Source: CAD feature listing. Evaluate the final solid. Frame: model axes, mm. A direction names the side the tool comes from. Give positions to 0.01 mm unless a question says otherwise; leave off trailing zeros. Loops run counter-clockwise (first coordinate to the right, second up) from the corner with the lowest first, then second, coordinate; pieces in that order, holes last. Notation, with made-up numbers: (-16.5, 25.25) -> (34.5, 25.25) arc R21 ccw to (34.5, 61.25) -> close; hole circle Ø9 at (-23.5, 60.25). An arc over 180 degrees is marked (long way). Put each result on its own line as item: value.
Autodesk Inventor part; units mm, degrees
ref_plane "YZ Plane" through (0, 0, 0) normal (1, 0, 0) x (0, 1, 0)
ref_plane "XZ Plane" through (0, 0, 0) normal (0, 1, 0) x (-1, 0, 0)
ref_plane "XY Plane" through (0, 0, 0) normal (0, 0, 1) x (1, 0, 0)
sketch "Sketch2" plane through (0, 0, 0) normal (0, 0, 1) x (1, 0, 0)
  circle A0 centre (0, 0) radius 14
  dimension "d1" = 28
extrude "Extrusion1" add sketch "Sketch2" along normal mid plane 30
sketch "Sketch3" plane through (0, 0, 15) normal (0, 0, 1) x (1, 0, 0)
  point P0 (0, 0)
hole "Hole1" at (0, 0, 15) direction (0, 0, -1) diameter 3.2 depth 5
sketch "Sketch4" plane through (0, 0, 10) normal (0, 0, 1) x (1, 0, 0)
  circle A0 centre (0, 0) radius 1.6
  line L0 (-1.5877, 2.75) -> (1.5877, 2.75)
  line L1 (1.5877, 2.75) -> (3.1754, 0)
  line L2 (3.1754, 0) -> (1.5877, -2.75)
  line L3 (1.5877, -2.75) -> (-1.5877, -2.75)
  line L4 (-1.5877, -2.75) -> (-3.1754, 0)
  line L5 (-3.1754, 0) -> (-1.5877, 2.75)
  dimension "d11" = 5.5
extrude "Extrusion2" cut sketch "Sketch4" against normal up to surface (10 mm away) contours A0 | L0 L1 L2 L3 L4 L5
sketch "Sketch5" plane through (0, 0, -15) normal (0, 0, -1) x (-1, 0, 0)
  circle A0 centre (0, 0) radius 2.5
  line L0 (-1.5, 2) -> (1.5, 2)
  dimension "d41" = 5
  dimension "d42" = 4.5
extrude "Extrusion3" cut sketch "Sketch5" against normal up to surface (15 mm away) contours A0 L0 picked at (0.1119, 0.5076)
sketch "Sketch8" plane through (0, 0, 0) normal (1, 0, 0) x (0, 1, 0)
  line L0 (2.85, 0) -> (-2.85, 0)
  line L1 (-2.85, 0) -> (-2.85, 2.6)
  line L2 (-2.85, 2.6) -> (2.85, 2.6)
  line L3 (2.85, 2.6) -> (2.85, 0)
  point P0 (0, 0)
  dimension "d48" = 2.6
  dimension "d49" = 5.7
extrude "Extrusion4" cut sketch "Sketch8" along normal through all both and the other way through all
equation "\"d30\" = 55deg"
equation "\"Sketch6_Pitch\" = 1.25"
properties part number "DestinationSpoolHolder"
(1) Line query: probe 1 along Z at (x, y) = (11, -2.75); probe 2 along X at (y, z) = (0, 13). Output: solid intervals per line, ascending. Write a range as from..to.
Calculated:
probe 1: z = -15..0, 2.6..15
probe 2: x = -14..-1.6, 1.6..14
(2) First-contact query: P1, Ø2, axis at y = 9, z = -4.5, coming from the +X side; P2, Ø12, axis at y = -7, z = 1.5, coming from the -X side; P3, Ø1, axis at x = 1.5, z = -2.5, coming from the +Y side; P4, Ø2.5, axis at x = 0, y = 0, coming from the +Z side. Flat tips, straight axial feed; report the tip coordinate or a pass-through.
Calculated:
P1: stops at x = 11.49
P2: stops at x = -13.96
P3: stops at y = 13.96
P4: passes through
(3) Section A-A on z = 8.5. Return loops of the section in (x, y).
Calculated:
outline: circle Ø28 at (0, 0); hole (-3.18, 0) -> (-1.59, -2.75) -> (1.59, -2.75) -> (3.18, 0) -> (1.59, 2.75) -> (-1.59, 2.75) -> close
(4) Draft query along Y for faces 1 (the flat face through (0, -2.75, 6)), 2 (the flat face through (0, -3, -15)), 3 (the cylindrical face through (13.35, 4.21, 0.21)). Return one class per face: released by +Y, released by -Y, zero draft, split by the parting line, or undercut.
Calculated:
face 1: undercut
face 2: zero draft
face 3: split by the parting line
(5) Section C-C on x = 4.25. Return loops of the section in (y, z).
Calculated:
outline: (-13.34, -15) -> (13.34, -15) -> (13.34, 15) -> (-13.34, 15) -> close; hole (-2.85, 0) -> (2.85, 0) -> (2.85, 2.6) -> (-2.85, 2.6) -> close
(6) Reachability of faces 4 (the cylindrical face through (0.1, -2.5, -7.6)), 5 (the flat face through (2.39, -1.36, 6.35)), 6 (the flat face through (0, 2.85, 1)) from +Z, -Z, +X, -X, +Y, -Y: full face, straight path, thin tool, end or side. Return the list, or none.
Calculated:
face 4: -Z
face 5: none
face 6: +X, -X
(7) Section D-D on y = -3.25. Return loops of the section in (x, z), then the cut area to 3 significant figures.
Calculated:
outline: (-13.62, -15) -> (13.62, -15) -> (13.62, 15) -> (-13.62, 15) -> close
area: 817 mm²
(8) Section B-B on x = 0. Return loops of the section in (y, z).
Calculated:
outline: (-14, -15) -> (-2.5, -15) -> (-2.5, 0) -> (-2.85, 0) -> (-2.85, 2.6) -> (-2.75, 2.6) -> (-2.75, 10) -> (-1.6, 10) -> (-1.6, 15) -> (-14, 15) -> close; (1.6, 10) -> (2.75, 10) -> (2.75, 2.6) -> (2.85, 2.6) -> (2.85, 0) -> (2, 0) -> (2, -15) -> (14, -15) -> (14, 15) -> (1.6, 15) -> close
